Autodesk Inventor part; units mm, degrees
ref_plane "YZ Plane" through (0, 0, 0) normal (1, 0, 0) x (0, 1, 0)
ref_plane "XZ Plane" through (0, 0, 0) normal (0, 1, 0) x (-1, 0, 0)
ref_plane "XY Plane" through (0, 0, 0) normal (0, 0, 1) x (1, 0, 0)
sketch "Sketch1" plane through (0, 0, 0) normal (0, 1, 0) x (-1, 0, 0)
  line L0 (0, 0) -> (-25, 0)
  line L1 (-25, 0) -> (-25, -25)
  line L2 (-25, -25) -> (0, -25)
  line L3 (0, -25) -> (0, 0)
  dimension "d0" = 25
  dimension "d1" = 25
extrude "Extrusion1" add sketch "Sketch1" along normal blind 5
sketch "Sketch2" plane through (0, 5, 0) normal (0, 1, 0) x (1, 0, 0)
  line L0 (25, 0) -> (25, 25)
  line L1 (0, 0) -> (25, 0)
  line L2 (25, 0) -> (25, 7)
  line L3 (25, 7) -> (0, 7)
  line L4 (0, 7) -> (0, 0)
  dimension "d4" = 7
extrude "Extrusion2" add sketch "Sketch2" along normal blind 40
fillet "Fillet1" radius 3 1 edges at (12.5, 5, -7)
fillet "Fillet2" radius 4 1 edges at (25, 45, -3.5)
fillet "Fillet3" radius 4 1 edges at (0, 45, -3.5)
fillet "Fillet4" radius 4 2 edges at (25, 2.5, -25) (0, 2.5, -25)
properties part number "Support1"
The model under review builds one solid part; all positions refer to its coordinate system, in mm. A direction names the side the tool comes from. Give positions to 0.01 mm unless a question says otherwise; leave off trailing zeros. Write each loop counter-clockwise with the first axis right and the second up, starting at its lowest first coordinate (ties: lowest second). Pieces come first, ordered by that corner, then holes. Notation, with made-up numbers: (80, -35) -> (114, -35) arc R20 ccw to (114, -13) -> close; hole circle Ø9 at (16.5, 67.25). An arc over 180 degrees is marked (long way). Put each result on its own line as item: value.
(1) Tool access review of faces 1 (the flat face through (13, 26, -7)), 2 (the flat face through (13, 0, -12)): name each direction out of +Z, -Z, +X, -X, +Y, -Y from which nothing blocks a thin tool from reaching the whole face with its end or side.
Results are:
face 1: -Z, +X, -X, +Y
face 2: +Z, -Z, +X, -X, -Y
(2) We need section C-C, the plane y = 22. Give the boundary of the cut face in (x, z), and give its area (3 significant figures).
Results are:
outline: (0, -7) -> (25, -7) -> (25, 0) -> (0, 0) -> close
area: 175 mm²
(3) We need section D-D, the plane x = 22.5. Give the boundary of the cut face in (y, z), and give its area (3 significant figures).
Results are:
outline: (0, -24.71) -> (5, -24.71) -> (5, -10) arc R3 cw to (8, -7) -> (44.71, -7) -> (44.71, 0) -> (0, 0) -> close
area: 403 mm²
(4) We need section A-A, the plane x = 19.25. Give the boundary of the cut face in (y, z).
Results are:
outline: (0, -25) -> (5, -25) -> (5, -10) arc R3 cw to (8, -7) -> (45, -7) -> (45, 0) -> (0, 0) -> close
(5) To check wall thickness, follow probe 1 along Y at (x, z) = (12.75, -14); probe 2 along Z at (x, y) = (13.5, 30); probe 3 along Z at (x, y) = (7, 6.5). State the ranges of each line that lie inside material, in increasing order. Write a range as from..to.
Results are:
probe 1: 0..5
probe 2: -7..0
probe 3: -7.4..0
(6) For pin 1 Ø1.5 at (x, y) = (3.5, 6.5) entering from +Z; pin 2 Ø12.5 at (x, y) = (11.5, 21.5) entering from -Z; pin 3 Ø12 at (y, z) = (32.5, -17) entering from -X, all flat-tipped, find the tip position at first contact; note any pin that passes through.
Results are:
pin 1: z = 0
pin 2: z = -7
pin 3: through
(7) We need section B-B, the plane z = -17.5. Give the boundary of the cut face in (x, y), and give its area (3 significant figures).
Results are:
outline: (0, 0) -> (25, 0) -> (25, 5) -> (0, 5) -> close
area: 125 mm²
